Model file for the job. Use its own axes, mm. Round coordinates to 2 decimals unless told otherwise and drop trailing zeros. Order: outer loops, then holes, each group sorted by start corner. A loop starts at its lowest first (then second) coordinate and runs counter-clockwise, first axis right, second up. Notation, with made-up numbers: (-32, -9) -> (-19, -9) arc R28 cw to (-19, 11) -> close; hole circle Ø9 at (-7, 44.25). An arc over 180 degrees is marked (long way). Answer as CSV lines item,"result".
Solid Edge part; units mm, degrees
sketch "Sketch1" plane through (0, 0, 0) normal (1, 0, 0) x (0, 1, 0)
  line L0 (-25, -11) -> (25, -11)
  line L1 (25, -11) -> (25, 11)
  line L2 (25, 11) -> (-25, 11)
  line L3 (-25, 11) -> (-25, -11)
extrude "Protrusion1" add sketch "Sketch1" against normal blind 3
sketch "Sketch2" plane through (-1.5, 0, 11) normal (0, 0, 1) x (0, 1, 0)
  circle A0 centre (-23, 0) radius 1.25
  circle A1 centre (-19.1667, 0) radius 1.25
  circle A2 centre (-15.3333, 0) radius 1.25
  circle A3 centre (-11.5, 0) radius 1.25
  circle A4 centre (-7.6667, 0) radius 1.25
  circle A5 centre (-3.8333, 0) radius 1.25
  circle A6 centre (0, 0) radius 1.25
  circle A7 centre (3.8333, 0) radius 1.25
  circle A8 centre (7.6667, 0) radius 1.25
  circle A9 centre (11.5, 0) radius 1.25
  circle A10 centre (15.3333, 0) radius 1.25
  circle A11 centre (19.1667, 0) radius 1.25
  circle A12 centre (23, 0) radius 1.25
extrude "ExtrudedCutout_49" cut sketch "Sketch2" against normal blind 6
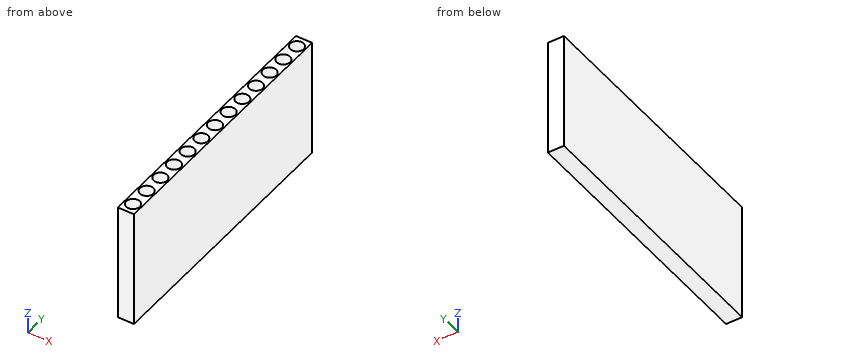
Q1. Saw through at C-C (y = -11). Write the cut outline in (x, z), plus the area to 3 significant figures.
Checks:
outline,"(-3, -11) -> (0, -11) -> (0, 11) -> (-0.35, 11) -> (-0.35, 5) -> (-2.65, 5) -> (-2.65, 11) -> (-3, 11) -> close"
area,"52.3 mm²"
Q2. Wall check: L1, parallel to X at y = 0, z = 8.4; L2, parallel to Z at x = -1.5, y = -22.5; L3, parallel to X at y = -20, z = 7.25. Give the ranges that are in metal, low to high. Write a range as [from, to].
Checks:
L1,"[-3, -2.75], [-0.25, 0]"
L2,"[-11, 5]"
L3,"[-3, -2.43], [-0.57, 0]"
Q3. Saw through at A-A (z = 6). State how many separate pieces and enclosed holes the cut face has, plus the area to 3 significant figures.
Checks:
separate pieces,"1"
enclosed holes,"13"
area,"86.2 mm²"
Q4. Saw through at B-B (y = 11.5). Write the cut outline in (x, z), plus the area to 3 significant figures.
Checks:
outline,"(-3, -11) -> (0, -11) -> (0, 11) -> (-0.25, 11) -> (-0.25, 5) -> (-2.75, 5) -> (-2.75, 11) -> (-3, 11) -> close"
area,"51.0 mm²"
Q5. Flat gauge pin, fed straight in: pin 1 (0.8 mm diameter, centred on x = -1, y = -19, fed in from +Z). Where does the tip first touch, or does it go through?
Checks:
pin 1,"z = 5"
